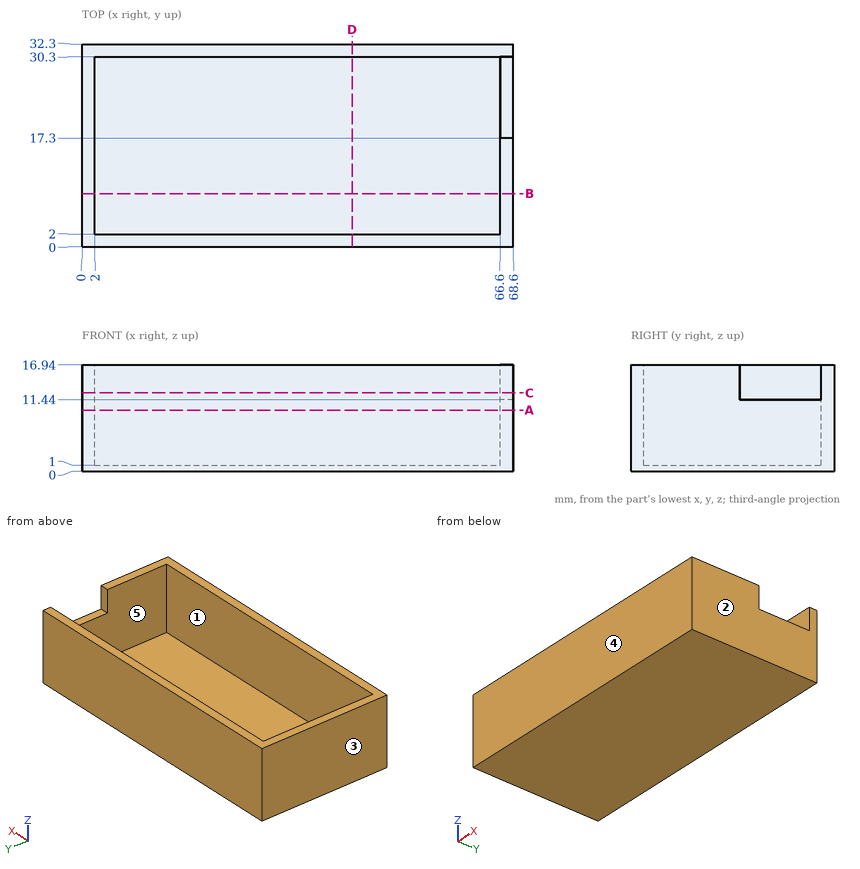
Check sheet for the drawn part. Datum: minimum x, y, z corner. Units: mm. A direction names the side the tool comes from. Round coordinates to 2 decimals unless told otherwise and drop trailing zeros. Order: outer loops, then holes, each group sorted by start corner. A loop starts at its lowest first (then second) coordinate and runs counter-clockwise, first axis right, second up. Notation, with made-up numbers: M 16,47.25 L 58,47.25 A15 ccw 58,54.25 Z; hole C 61.25,47 d9. An arc over 180 degrees is marked long. Answer in a Markdown table with one row per item.
(1) Section check C-C on z = 12.5. Record the boundary of the cut face in (x, y), plus the area to 3 significant figures.
Findings:
| item | result |
|---|---|
| outline | M 0,0 L 68.6,0 L 68.6,17.3 L 66.6,17.3 L 66.6,2 L 2,2 L 2,30.3 L 68.6,30.3 L 68.6,32.3 L 0,32.3 Z |
| area | 362 mm^2 |
(2) Material ranges on line 1 along Y through (x, z) = (53, 14); line 2 along X through (y, z) = (12, 13.75); line 3 along Z through (x, y) = (63, 24), recorded low to high. Write a range as from..to.
Findings:
| item | result |
|---|---|
| line 1 | y = 0..2, 30.3..32.3 |
| line 2 | x = 0..2, 66.6..68.6 |
| line 3 | z = 0..1 |
(3) Section check A-A on z = 9.75. Record the boundary of the cut face in (x, y), plus the area to 3 significant figures.
Findings:
| item | result |
|---|---|
| outline | M 0,0 L 68.6,0 L 68.6,32.3 L 0,32.3 Z; hole M 2,2 L 66.6,2 L 66.6,30.3 L 2,30.3 Z |
| area | 388 mm^2 |
(4) Section check B-B on y = 8.5. Record the boundary of the cut face in (x, z).
Findings:
| item | result |
|---|---|
| outline | M 0,0 L 68.6,0 L 68.6,16.94 L 66.6,16.94 L 66.6,1 L 2,1 L 2,16.94 L 0,16.94 Z |
(5) Section check D-D on x = 43. Record the boundary of the cut face in (y, z), plus the area to 3 significant figures.
Findings:
| item | result |
|---|---|
| outline | M 0,0 L 32.3,0 L 32.3,16.94 L 30.3,16.94 L 30.3,1 L 2,1 L 2,16.94 L 0,16.94 Z |
| area | 96.1 mm^2 |
(6) Set-up check for the marked faces 1 and 2: record each of +Z, -Z, +X, -X, +Y, -Y from which the full face is reachable in a straight line by a thin tool's end or side.
Findings:
| item | result |
|---|---|
| face 1 | +Z |
| face 2 | +Z, -Z, +X, +Y, -Y |
(7) Gauge pin test, flat ends, axial feed: pin 1 (14 mm diameter, centred on x = 36.5, y = 10.5, fed in from +Z); pin 2 (1 mm diameter, centred on x = 67.5, y = 21.5, fed in from +Z). Record the tip position at first contact, or that the pin passes through.
Findings:
| item | result |
|---|---|
| pin 1 | stops at z = 1 |
| pin 2 | stops at z = 11.44 |
(8) Draft check along Y on the marked faces 3, 4 and 5. Enter one of: +Y half, -Y half, draft (parallel to the pull), parting line (faces both ways), or undercut.
Findings:
| item | result |
|---|---|
| face 3 | draft |
| face 4 | -Y half |
| face 5 | undercut |
